Model file for the job. Use its own axes, mm. Face numbers are marked on the shaded views. A direction names the side the tool comes from. Coordinates: 2 decimals unless noted, no trailing zeros. Order: outer loops, then holes, each group sorted by start corner. A loop starts at its lowest first (then second) coordinate and runs counter-clockwise, first axis right, second up.
from build123d import *

# Parameters (mm, degrees)
SKETCH2_R           = 9
BOSS_EXTRUDE1_DEPTH = 25
SKETCH3_R           = 6
BOSS_EXTRUDE2_DEPTH = 15
BOSS_EXTRUDE4_START = 15
SKETCH4_R           = 6
BOSS_EXTRUDE4_DEPTH = 15
SKETCH5_R           = 3
CUT_EXTRUDE1_DEPTH  = 10
SKETCH6_R           = 3
CUT_EXTRUDE2_DEPTH  = 45
CHAMFER1_SIZE       = 1
CHAMFER2_SIZE       = 1


with BuildPart() as part:
    # Sketch2 → Boss-Extrude1 (new, symmetric)
    with BuildSketch(Plane.XY):
        Circle(SKETCH2_R)
    extrude(amount=BOSS_EXTRUDE1_DEPTH, both=True)

    # Sketch3 → Boss-Extrude2 (add)
    with BuildSketch(Plane.XY.offset(25)):
        Circle(SKETCH3_R)
    extrude(amount=BOSS_EXTRUDE2_DEPTH)

    # Sketch4 → Boss-Extrude4 (add)
    with BuildSketch(Plane(origin=(0, 0, -25), x_dir=(-1, 0, 0), z_dir=(0, 0, -1)).offset(BOSS_EXTRUDE4_START)):
        with Locations(Location((0, 0, 0), (0, 0, 180))):
            Circle(SKETCH4_R)
    extrude(amount=-BOSS_EXTRUDE4_DEPTH)

    # Sketch5 → Cut-Extrude1 (cut, symmetric)
    with BuildSketch(Plane(origin=(0, 0, 0), x_dir=(0, 0, -1), z_dir=(1, 0, 0))):
        with Locations(Location((0, 0, 0), (0, 0, 180))):
            Circle(SKETCH5_R)
    extrude(amount=CUT_EXTRUDE1_DEPTH, both=True, mode=Mode.SUBTRACT)

    # Sketch6 → Cut-Extrude2 (cut)
    with BuildSketch(Plane.XY.offset(40)):
        Circle(SKETCH6_R)
    extrude(amount=-CUT_EXTRUDE2_DEPTH, mode=Mode.SUBTRACT)

    # Sketch7 → Cut-Revolve1 (revolve, cut)
    with BuildSketch(Plane(origin=(0, 0, 0), x_dir=(1, 0, 0), z_dir=(0, 1, 0))):
        Polygon((-3, 5), (0, 8), (0, 5), align=None)
    revolve(axis=Axis((0, 0, -10.064608653), (0, 0, 1)), mode=Mode.SUBTRACT)

    # Chamfer1
    chamfer1_edges = [part.edges().sort_by_distance(p)[0] for p in [
        (-6, 0, 40),
    ]]
    chamfer(chamfer1_edges, length=CHAMFER1_SIZE)

    # Chamfer2
    chamfer2_edges = [part.edges().sort_by_distance(p)[0] for p in [
        (-6, 0, -40),
    ]]
    chamfer(chamfer2_edges, length=CHAMFER2_SIZE)


solid = part.part
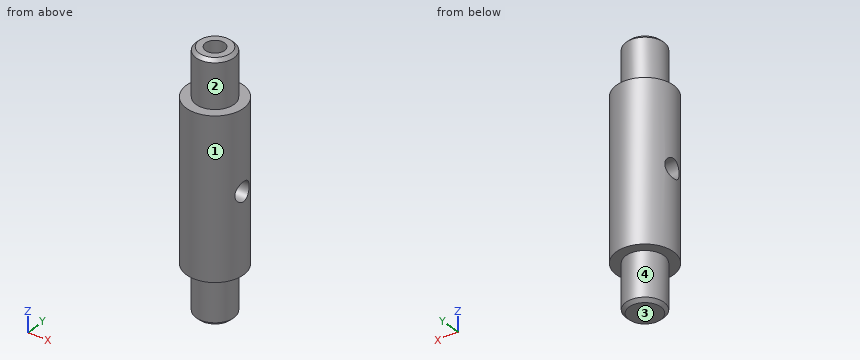
Q1. Cut at D-D, the plane z = -15. List the corners of the cut face in (x, y), plus the area to 3 significant figures.
Established:
outline: circle Ø18 at (0, 0)
area: 254 mm2
Q2. Mould opens along X. For the marked faces 3 and 4 say: pulls with the +X half, pulls with the -X half, needs draft (parallel to the pull), parting line crosses it, or undercut.
Established:
face 3: needs draft
face 4: parting line crosses it
Q3. Cut at C-C, the plane z = 14. List the corners of the cut face in (x, y), plus the area to 3 significant figures.
Established:
outline: circle Ø18 at (0, 0); hole circle Ø6 at (0, 0)
area: 226 mm2
Q4. Drop flat-ended pins along their axis: P1, Ø5, axis at x = 0, y = 0, coming from the +Z side; P2, Ø1.5, axis at y = 5, z = -2.5, coming from the +X side; P3, Ø5, axis at x = 3.5, z = -2, coming from the -Y side; P4, Ø8, axis at x = -2, z = -17.5, coming from the -Y side. Give the stop position or say it passes through.
Established:
P1: stops at z = -5.5
P2: stops at x = 7.93
P3: stops at y = -8.94
P4: stops at y = -9
Q5. Cut at A-A, the plane z = 2. List the corners of the cut face in (x, y), plus the area to 3 significant figures.
Established:
outline: (-8.72, -2.24) arc R9 ccw to (8.72, -2.24) - (2, -2.24) arc R3 cw to (-2, -2.24) - close; (-8.72, 2.24) - (-2, 2.24) arc R3 cw to (2, 2.24) - (8.72, 2.24) arc R9 ccw to start
area: 171 mm2
Q6. Cut at B-B, the plane x = 7.5. List the corners of the cut face in (y, z), plus the area to 3 significant figures.
Established:
outline: (-4.97, -25) - (4.97, -25) - (4.97, 25) - (-4.97, 25) - close; hole circle Ø6 at (0, 0)
area: 469 mm2
Q7. Which spindle directions (+Z, -Z, +X, -X, +Y, -Y) get a long thin tool onto all of the face, cutting with end or side? Do the marked faces 1 and 2. Say none if no direction does.
Established:
face 1: +Z, -Z
face 2: +Z
Q8. Probe line 1 (X direction, y = 0, z = -3.9); line 2 (Z direction, x = 6.5, y = 5.25). List the from-to ranges inside material, lowest first.
Established:
line 1: x = -9 to -3, 3 to 9
line 2: z = -25 to 25
